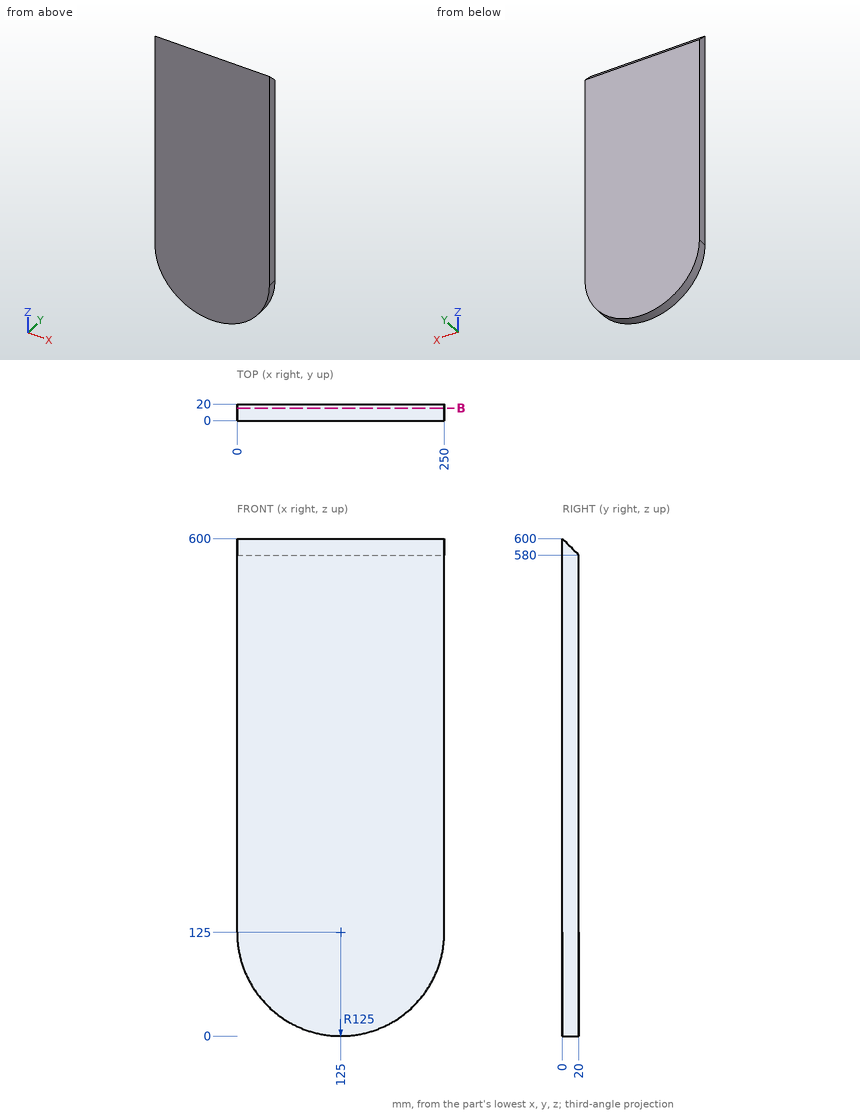
For this review, use the dimensioned drawing (mm, ordinates from the lowest corner) and the shaded views. Coordinates: 2 decimals unless noted, no trailing zeros. Write each loop counter-clockwise with the first axis right and the second up, starting at its lowest first coordinate (ties: lowest second). Pieces come first, ordered by that corner, then holes. Notation, with made-up numbers: (74, -1) - (122, -1) arc R20 ccw to (122, 15) - close; hole circle Ø3 at (14.25, 63.5). An arc over 180 degrees is marked (long way). Answer in a Markdown table with one row per item. Add a question column.
Q1. To check wall thickness, follow line 1 along X through (y, z) = (4, 92.5); line 2 along Z through (x, y) = (38, 10.25); line 3 along Z through (x, y) = (90.5, 14.5). State the ranges of each line that lie inside material, in increasing order. Write a range as from..to.
Q2. Clearance check with flat-ended pins moving along their axes: pin 1 (12 mm diameter, centred on y = 15, z = 378.5, fed in from -X); pin 2 (5 mm diameter, centred on x = 102, y = 13, fed in from +Z); pin 3 (6 mm diameter, centred on x = 52.5, y = 15, fed in from +Z); pin 4 (12 mm diameter, centred on x = 82, y = 15, fed in from -Z). State where each tip first meets the part, or that it passes through.
Q3. Consider section B-B on y = 15. Give the boundary of the cut face in (x, z), then the cut area to 3 significant figures.
Answers below:
| question | item | result |
|---|---|---|
| 1 | line 1 | 4.3..245.7 |
| 1 | line 2 | 35.24..589.75 |
| 1 | line 3 | 4.86..585.5 |
| 2 | pin 1 | x = 0 |
| 2 | pin 2 | z = 589.5 |
| 2 | pin 3 | z = 588 |
| 2 | pin 4 | z = 5.6 |
| 3 | outline | (0, 125) arc R125 ccw to (250, 125) - (250, 585) - (0, 585) - close |
| 3 | area | 140,000 mm² |
